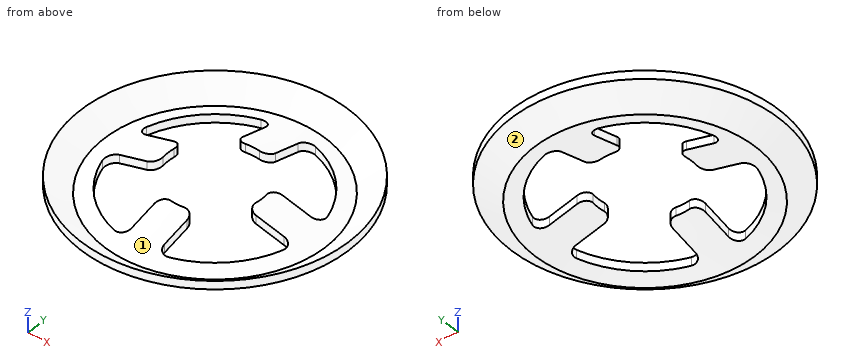
```python
from build123d import *

# Parameters (mm, degrees)
CUT_EXTRUDE1_DEPTH       = 6.669270235
FILLET1_R                = 0.25
CIRPATTERN1_COUNT        = 4
FILLET1_OF_CIRPATTERN1_R = 0.25


with BuildPart() as part:
    # Sketch2 → Revolve1 (revolve)
    with BuildSketch(Plane(origin=(0, 0, 0), x_dir=(0, 0, -1), z_dir=(1, 0, 0)), mode=Mode.PRIVATE) as revolve1_sk:
        Polygon((-0.375, 4), (0.125, 3.3), (-0.375, 1.4), (-0.125, 1.4), (0.375, 3.3), (-0.125, 4), align=None)
    revolve(revolve1_sk.sketch.rotate(Axis((0, 0, 0.375), (0, 0, -1)), 90), axis=Axis((0, 0, 0.375), (0, 0, -1)))

    # Sketch3 → Cut-Extrude1 (cut, symmetric)
    with BuildSketch(Plane.XY):
        with BuildLine():
            Line((-0.490556102, 2.782081902), (-0.490556102, 0.490556102))
            Line((-0.490556102, 0.490556102), (-2.782081902, 0.490556102))
            ThreePointArc((-2.782081902, 0.490556102), (-1.997576657, 1.997576657), (-0.490556102, 2.782081902))
        make_face()
    cut_extrude1 = extrude(amount=CUT_EXTRUDE1_DEPTH, both=True, mode=Mode.SUBTRACT)

    # Fillet1
    fillet1_edges = [part.edges().sort_by_distance(p)[0] for p in [
        (-1.311241668, 0.490556102, 0.25),
        (-0.490556102, 1.311241668, 0.25),
        (-2.782081902, 0.490556102, -0.125),
        (-0.490556102, 2.782081902, -0.125),
    ]]
    fillet(fillet1_edges, radius=FILLET1_R)

    # CirPattern1: Cut-Extrude1 ×4 about axis
    cirpattern1_axis = Axis((0, 0, 0), (0, 0, 1))
    for i in range(1, CIRPATTERN1_COUNT):
        add(cut_extrude1.rotate(cirpattern1_axis, i * 360 / CIRPATTERN1_COUNT), mode=Mode.SUBTRACT)

    # Fillet1 of CirPattern1
    fillet1_of_cirpattern1_edges = [part.edges().sort_by_distance(p)[0] for p in [
        (-0.490556102, -1.311241668, 0.25),
        (-1.311241668, -0.490556102, 0.25),
        (-0.490556102, -2.782081902, -0.125),
        (-2.782081902, -0.490556102, -0.125),
        (1.311241668, -0.490556102, 0.25),
        (0.490556102, -1.311241668, 0.25),
        (2.782081902, -0.490556102, -0.125),
        (0.490556102, -2.782081902, -0.125),
        (0.490556102, 1.311241668, 0.25),
        (1.311241668, 0.490556102, 0.25),
        (0.490556102, 2.782081902, -0.125),
        (2.782081902, 0.490556102, -0.125),
    ]]
    fillet(fillet1_of_cirpattern1_edges, radius=FILLET1_OF_CIRPATTERN1_R)


solid = part.part
```
Could you check a few things on this model? Use its own coordinates, in mm. Face numbers are marked on the shaded views. Round coordinates to 2 decimals unless told otherwise and drop trailing zeros. Loops run counter-clockwise (first coordinate to the right, second up) from the corner with the lowest first, then second, coordinate; pieces in that order, holes last.
Q1. Please list where these lines run through material, in increasing order: L1, parallel to X at y = -1.5, z = 0.2; L2, parallel to Y at x = 1.75, z = -0.2; L3, parallel to X at y = 2.75, z = 0.25.
Q2. For P1, Ø4, axis at x = -2, y = 1.5, coming from the -Z side (3 decimals), with a flat end and sliding along its axis, tell me the tip position at first contact or that it passes through.
Q3. I want a section at A-A (y = 0). Write out the boundary of the cut face in (x, z) (3 decimals), and give its area (3 significant figures).
Q4. I want a section at C-C (y = 2.25). Give the number of separate pieces and of enclosed holes in the cut face, and give its area (3 significant figures).
Q5. Thinking about a two-plate mould opening in X: for the marked faces 1 and 2, which applies, pulls with the +X half, pulls with the -X half, needs draft (parallel to the pull), parting line crosses it, or undercut?
Answer below:
1. L1: x = -3.71 to -3.44, -0.45 to 0.45, 3.44 to 3.71
1. L2: y = -3.08 to -2.22, 2.22 to 3.08
1. L3: x = -2.9 to -2.66, 2.66 to 2.9
2. P1: stops at z = -0.375
3. outline: (-4, 0.125) - (-3.3, -0.375) - (-1.4, 0.125) - (-1.4, 0.375) - (-3.3, -0.125) - (-4, 0.375) - close; (1.4, 0.125) - (3.3, -0.375) - (4, 0.125) - (4, 0.375) - (3.3, -0.125) - (1.4, 0.375) - close
3. area: 1.30 mm2
4. separate pieces: 3
4. enclosed holes: 0
4. area: 1.04 mm2
5. face 1: undercut
5. face 2: parting line crosses it
